Part model, mm, in its own coordinate system. A direction names the side the tool comes from. Round coordinates to 2 decimals unless told otherwise and drop trailing zeros. Write each loop counter-clockwise with the first axis right and the second up, starting at its lowest first coordinate (ties: lowest second). Pieces come first, ordered by that corner, then holes. Notation, with made-up numbers: (2, 27) -> (45, 27) arc R10 cw to (45, 33) -> close; hole circle Ø1 at (75, 4.5). An arc over 180 degrees is marked (long way). Return JSON: item names as keys, results as strings. Group by question number.
```python
from build123d import *

# Parameters (mm, degrees)
SKETCH2_W           = 28.40399364
SKETCH2_H           = 29.4
BOSS_EXTRUDE1_DEPTH = 30.48
BOSS_EXTRUDE2_DEPTH = 3.48
SKETCH7_W           = 14.151447967
SKETCH7_H           = 4.326095682
BOSS_EXTRUDE3_DEPTH = 30.48
SKETCH8_R           = 1.986850399
CUT_EXTRUDE3_DEPTH  = 4.48
FILLET2_R           = 10
SKETCH4_R           = 2.85648699
CUT_EXTRUDE2_DEPTH  = 30.48
FILLET3_R           = 10
SKETCH9_R           = 1.75
CUT_EXTRUDE4_DEPTH  = 4.48
SKETCH3_W           = 26.67
SKETCH3_H           = 26.67
CUT_EXTRUDE1_DEPTH  = 30.48
FILLET4_R           = 10


with BuildPart() as part:
    # Sketch2 → Boss-Extrude1 (new body)
    with BuildSketch(Plane.XY):
        with Locations((48.284161423, 4.792820272)):
            Rectangle(SKETCH2_W, SKETCH2_H)
    extrude(amount=BOSS_EXTRUDE1_DEPTH)

    # Sketch5 → Boss-Extrude2 (add)
    with BuildSketch(Plane(origin=(0, 0, 0), x_dir=(-1, 0, 0), z_dir=(0, 0, -1))):
        Polygon((-62.486158243, 19.492820272), (-62.486158243, 65.492820272), (-48.334710276, 65.492820272), (-34.082164603, 19.492820272), align=None)
    boss_extrude2 = extrude(amount=-BOSS_EXTRUDE2_DEPTH)

    # Sketch7 → Boss-Extrude3 (add)
    with BuildSketch(Plane(origin=(0, 0, 0), x_dir=(-1, 0, 0), z_dir=(0, 0, -1))):
        with Locations((-55.41043426, 63.329772431)):
            Rectangle(SKETCH7_W, SKETCH7_H)
    boss_extrude3 = extrude(amount=BOSS_EXTRUDE3_DEPTH)

    # Sketch8 → Cut-Extrude3 (cut)
    with BuildSketch(Plane(origin=(0, 65.492820272, 0), x_dir=(1, 0, 0), z_dir=(0, 1, 0))):
        with Locations(Location((58.338019211, 18.1, 0), (0, 0, 270))):
            Circle(SKETCH8_R)
    extrude(amount=-CUT_EXTRUDE3_DEPTH, mode=Mode.SUBTRACT)

    # Fillet2
    fillet2_edges = [part.edges().sort_by_distance(p)[0] for p in [
        (48.284161423, 19.492820272, 3.48),
    ]]
    fillet(fillet2_edges, radius=FILLET2_R)

    # Mirror3: Boss-Extrude2, Boss-Extrude3 across plane
    add(boss_extrude2.mirror(Plane(origin=(0, 4.792820272, 0), x_dir=(0, 0, 1), z_dir=(0, -1, 0))))
    add(boss_extrude3.mirror(Plane(origin=(0, 4.792820272, 0), x_dir=(0, 0, 1), z_dir=(0, -1, 0))))

    # Sketch4 → Cut-Extrude2 (cut)
    with BuildSketch(Plane.XY.offset(30.48)):
        with Locations((47.902483521, 4.05454278)):
            Circle(SKETCH4_R)
    extrude(amount=-CUT_EXTRUDE2_DEPTH, mode=Mode.SUBTRACT)

    # Fillet3
    fillet3_edges = [part.edges().sort_by_distance(p)[0] for p in [
        (48.284161423, -9.907179728, 3.48),
    ]]
    fillet(fillet3_edges, radius=FILLET3_R)

    # Sketch9 → Cut-Extrude4 (cut)
    with BuildSketch(Plane.XZ.offset(55.907179728)):
        with Locations(Location((58.338019211, -18.1, 0), (0, 0, 270))):
            Circle(SKETCH9_R)
    extrude(amount=-CUT_EXTRUDE4_DEPTH, mode=Mode.SUBTRACT)

    # Sketch3 → Cut-Extrude1 (cut)
    with BuildSketch(Plane(origin=(62.486158243, 0, 0), x_dir=(0, 0, -1), z_dir=(1, 0, 0))):
        with Locations((-15.72499675, 4.792820272)):
            Rectangle(SKETCH3_W, SKETCH3_H)
    extrude(amount=-CUT_EXTRUDE1_DEPTH, mode=Mode.SUBTRACT)

    # Fillet4
    fillet4_edges = [part.edges().sort_by_distance(p)[0] for p in [
        (48.334710276, 63.329772431, -30.48),
        (48.334710276, -53.744131887, -30.48),
    ]]
    fillet(fillet4_edges, radius=FILLET4_R)


solid = part.part
```
Item 1: Cut at A-A (z = -18.1). Write the cut outline in (x, y).
Item 2: Cut at C-C (x = 46.5). Write the cut outline in (y, z).
Item 3: Cut at D-D (y = 53). Write the cut outline in (x, z).
Item 4: Two-plate mould, pull along Y, no slides. Class faces 1 (the face through (48, 8, 29.06)), 2 (the face through (40.714, -31.311, 2.215)), 3 (the face through (48.335, -54, -10)): released by +Y, released by -Y, zero draft, split by the parting line, or undercut.
Item 5: Cut at B-B (z = 5.5). Write the cut outline in (x, y), then the cut area to 3 significant figures.
Item 6: Wall check: L1, parallel to Z at x = 56.75, y = -4.5; L2, parallel to Y at x = 41, z = 26.5; L3, parallel to Y at x = 56.25, z = -5. Give the ranges that are in metal, low to high.
Item 7: Flat gauge pins, fed straight in: P1, Ø1.3, axis at y = -53.5, z = -8.5, coming from the -X side; P2, Ø8.5, axis at x = 48, y = 10, coming from the -Z side; P3, Ø3, axis at x = 55.5, y = 35, coming from the +Z side; P4, Ø3.5, axis at x = 47.9, y = 4.05, coming from the +Z side. Where does each tip first touch, or does it go through?
Item 8: Which spindle directions (+Z, -Z, +X, -X, +Y, -Y) get a long thin tool onto all of the face, cutting with end or side? Do faces 4 (the face through (56, -51.581, -15)), 5 (the face through (48, -8.542, 16)), 6 (the face through (52, -38, 3.48)), 7 (the face through (48, 19.493, 22)), 8 (the face through (48.335, 63, -10)). Say none if no direction does.
Checks:
{
 "1": {"outline": "(48.33, -55.91) -> (56.59, -55.91) -> (56.59, -51.58) -> (48.33, -51.58) -> close; (48.33, 61.17) -> (56.35, 61.17) -> (56.35, 65.49) -> (48.33, 65.49) -> close; (60.09, -55.91) -> (62.49, -55.91) -> (62.49, -51.58) -> (60.09, -51.58) -> close; (60.32, 61.17) -> (62.49, 61.17) -> (62.49, 65.49) -> (60.32, 65.49) -> close"},
 "2": {"outline": "(-49.99, 0) -> (1.57, 0) -> (1.57, 2.39) -> (-8.54, 2.39) -> (-8.54, 29.06) -> (1.57, 29.06) -> (1.57, 30.48) -> (-9.91, 30.48) -> (-9.91, 13.48) arc R10 cw to (-19.91, 3.48) -> (-49.99, 3.48) -> close; (6.54, 0) -> (59.57, 0) -> (59.57, 3.48) -> (29.49, 3.48) arc R10 cw to (19.49, 13.48) -> (19.49, 30.48) -> (6.54, 30.48) -> (6.54, 29.06) -> (18.13, 29.06) -> (18.13, 2.39) -> (6.54, 2.39) -> close"},
 "3": {"outline": "(44.46, 0) -> (62.49, 0) -> (62.49, 3.48) -> (44.46, 3.48) -> close"},
 "4": {"face 1": "undercut", "face 2": "released by -Y", "face 3": "zero draft"},
 "5": {"outline": "(34.08, -9.91) -> (35.31, -13.88) -> (62.49, -13.88) -> (62.49, -8.54) -> (34.08, -8.54) -> close; (34.08, 18.13) -> (62.49, 18.13) -> (62.49, 23.47) -> (35.31, 23.47) -> (34.08, 19.49) -> close", "area": "298 mm2"},
 "6": {"L1": "z = 0 to 2.39, 29.06 to 30.48", "L2": "y = -9.91 to -8.54, 18.13 to 19.49", "L3": "y = -55.91 to -51.58, 61.17 to 65.49"},
 "7": {"P1": "stops at x = 48.33", "P2": "stops at z = 0", "P3": "stops at z = 3.48", "P4": "passes through"},
 "8": {"face 4": "-Z, +X, -X", "face 5": "+X, -X", "face 6": "+Z, +X, -X, -Y", "face 7": "+Z, +X, -X, +Y", "face 8": "-Z, -X, +Y, -Y"}
}
